```python
from build123d import *

# Parameters (mm, degrees)
ESQUISSE1_W                  = 40
ESQUISSE1_H                  = 85
BOSS_EXTRU_1_DEPTH           = 45
ESQUISSE2_W                  = 38.25
ESQUISSE2_H                  = 38.25
ENL_V_MAT_EXTRU_1_DEPTH      = 41.1
ESQUISSE3_W                  = 42
ESQUISSE3_H                  = 22
ENL_V_MAT_EXTRU_2_DEPTH      = 105.16333328
ESQUISSE4_R                  = 18.25625
ENL_V_MAT_EXTRU_3_DEPTH      = 42
ENL_V_MAT_EXTRU_4_DEPTH      = 104.048532255
ENL_V_MAT_EXTRU_4_DEPTH_BACK = 104.048532255
ESQUISSE5_R                  = 11
ESQUISSE6_R                  = 1.625
ENL_V_MAT_EXTRU_5_DEPTH      = 103.902866821
ENL_V_MAT_EXTRU_6_DEPTH      = 103.75038017
ENL_V_MAT_EXTRU_6_DEPTH_BACK = 103.75038017
ESQUISSE7_R                  = 4.065
ESQUISSE8_W                  = 5
ESQUISSE8_H                  = 21.25625
ENL_V_MAT_EXTRU_7_DEPTH      = 105.16333328


with BuildPart() as part:
    # Esquisse1 → Boss.-Extru.1 (new body)
    with BuildSketch(Plane.XY):
        with Locations((20, 42.5)):
            Rectangle(ESQUISSE1_W, ESQUISSE1_H)
    extrude(amount=BOSS_EXTRU_1_DEPTH)

    # Esquisse2 → Enlèv. mat.-Extru.1 (cut)
    with BuildSketch(Plane(origin=(40, 0, 0), x_dir=(0, 0, -1), z_dir=(1, 0, 0))):
        with Locations((-22.5, 19.125)):
            Rectangle(ESQUISSE2_W, ESQUISSE2_H)
    extrude(amount=-ENL_V_MAT_EXTRU_1_DEPTH, mode=Mode.SUBTRACT)

    # Esquisse3 → Enlèv. mat.-Extru.2 (cut, through all)
    with BuildSketch(Plane(origin=(0, 0, 45), x_dir=(0, 0, -1), z_dir=(1, 0, 0))):
        with Locations((24, 74)):
            Rectangle(ESQUISSE3_W, ESQUISSE3_H)
    extrude(amount=ENL_V_MAT_EXTRU_2_DEPTH, mode=Mode.SUBTRACT)

    # Esquisse4 → Enlèv. mat.-Extru.3 (cut)
    with BuildSketch(Plane.XY):
        with Locations((20, 63)):
            Circle(ESQUISSE4_R)
    extrude(amount=ENL_V_MAT_EXTRU_3_DEPTH, mode=Mode.SUBTRACT)

    # Esquisse5 → Enlèv. mat.-Extru.4 (cut, two sides: drawn at the far end of the back side and taken through both)
    with BuildSketch(Plane(origin=(37, 0, 0), x_dir=(-1, 0, 0), z_dir=(0, 0, -1)).offset(-ENL_V_MAT_EXTRU_4_DEPTH_BACK)):
        with Locations((17, 63)):
            Circle(ESQUISSE5_R)
    extrude(amount=ENL_V_MAT_EXTRU_4_DEPTH + ENL_V_MAT_EXTRU_4_DEPTH_BACK, mode=Mode.SUBTRACT)

    # Esquisse6 → Enlèv. mat.-Extru.5 (cut, through all)
    with BuildSketch(Plane(origin=(0, 0, 42), x_dir=(-1, 0, 0), z_dir=(0, 0, -1))):
        with Locations((-29.545941546, 72.545941546)):
            Circle(ESQUISSE6_R)
        with Locations((-29.545941546, 52.545941546)):
            Circle(ESQUISSE6_R)
        with Locations((-9.545941546, 52.545941546)):
            Circle(ESQUISSE6_R)
        with Locations((-9.545941546, 72.545941546)):
            Circle(ESQUISSE6_R)
    extrude(amount=-ENL_V_MAT_EXTRU_5_DEPTH, mode=Mode.SUBTRACT)

    # Esquisse7 → Enlèv. mat.-Extru.6 (cut, two sides: drawn at the far end of the back side and taken through both)
    with BuildSketch(Plane(origin=(0, 0, 41.625), x_dir=(-1, 0, 0), z_dir=(0, 0, -1)).offset(-ENL_V_MAT_EXTRU_6_DEPTH_BACK)):
        with Locations((-10, 18.4875)):
            Circle(ESQUISSE7_R)
        with Locations((-30, 18.4875)):
            Circle(ESQUISSE7_R)
    extrude(amount=ENL_V_MAT_EXTRU_6_DEPTH + ENL_V_MAT_EXTRU_6_DEPTH_BACK, mode=Mode.SUBTRACT)

    # Esquisse8 → Enlèv. mat.-Extru.7 (cut, through all)
    with BuildSketch(Plane.ZY):
        with Locations((2.5, 52.371875)):
            Rectangle(ESQUISSE8_W, ESQUISSE8_H)
    extrude(amount=-ENL_V_MAT_EXTRU_7_DEPTH, mode=Mode.SUBTRACT)


solid = part.part
```
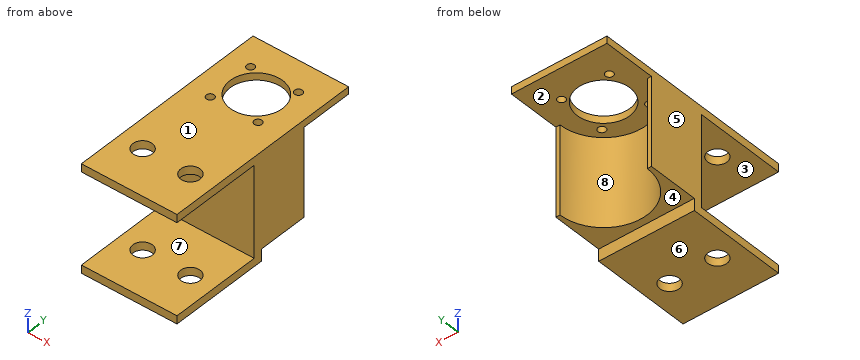
CAD build for the part. Positions are in the model's coordinates, mm. Face numbers are marked on the shaded views. A direction names the side the tool comes from. Coordinates: 2 decimals unless noted, no trailing zeros. Write each loop counter-clockwise with the first axis right and the second up, starting at its lowest first coordinate (ties: lowest second). Pieces come first, ordered by that corner, then holes. Notation, with made-up numbers: (65, 16.25) -> (78, 16.25) arc R30 cw to (78, 45.25) -> close; hole circle Ø4 at (49, 72). An arc over 180 degrees is marked (long way). Use CSV: the item, a comma, the result in double quotes. Start each with the question number.
Item 1: Drop flat-ended pins along their axis: P1, Ø8, axis at x = 11.5, y = 22, coming from the +Z side; P2, Ø8, axis at x = 29, z = 32, coming from the +Y side; P3, Ø12, axis at y = 72.5, z = 12, coming from the -X side; P4, Ø10.5, axis at x = 20.5, y = 49, coming from the -Z side. Give the stop position or say it passes through.
Item 2: Tool access for the marked faces 4, 5, 6, 7 and 8: list every direction of +Z, -Z, +X, -X, +Y, -Y with a clear straight run to the whole face (end or side of a thin tool).
Item 3: Band-saw the part on C-C, the plane x = 10. Give the number of separate pieces and of enclosed holes in the cut face, plus the area to 3 significant figures.
Item 4: Band-saw the part on D-D, the plane y = 20.5. Write the cut outline in (x, z) (3 decimals).
Item 5: Two-plate mould, pull along Z, no slides. Class the marked faces 1, 2 and 3: +Z half, -Z half, draft (parallel to the pull), parting line (faces both ways), or undercut.
Item 6: Band-saw the part on B-B, the plane y = 62. Write the cut outline in (x, z), plus the area to 3 significant figures.
Item 7: Band-saw the part on A-A, the plane x = 20. Write the cut outline in (y, z) (3 decimals), plus the area to 3 significant figures.
Item 8: Wall check: probe 1 along Z at (x, y) = (37.5, 34) (3 decimals); probe 2 along Y at (x, z) = (10, 0.9); probe 3 along Y at (x, z) = (20, 43). Give the ranges that are in metal, low to high.
Response values:
1,P1,"stops at z = 45"
1,P2,"stops at y = 50.18"
1,P3,"passes through"
1,P4,"stops at z = 5"
2,face 4,"-Z, +X, -X, +Y"
2,face 5,"+Z, -Z, -X, +Y, -Y"
2,face 6,"-Z, +X, -X, +Y, -Y"
2,face 7,"+X, -X, -Y"
2,face 8,"-Z, +Y"
3,separate pieces,"6"
3,enclosed holes,"0"
3,area,"665 mm2"
4,outline,"(0, 0) -> (6.468, 0) -> (6.468, 3.375) -> (0, 3.375) -> close; (0, 41.625) -> (6.468, 41.625) -> (6.468, 45) -> (0, 45) -> close; (13.532, 0) -> (26.468, 0) -> (26.468, 3.375) -> (13.532, 3.375) -> close; (13.532, 41.625) -> (26.468, 41.625) -> (26.468, 45) -> (13.532, 45) -> close; (33.532, 0) -> (40, 0) -> (40, 3.375) -> (33.532, 3.375) -> close; (33.532, 41.625) -> (40, 41.625) -> (40, 45) -> (33.532, 45) -> close"
5,face 1,"+Z half"
5,face 2,"-Z half"
5,face 3,"undercut"
6,outline,"(0, 5) -> (1.77, 5) -> (1.77, 42) -> (9.05, 42) -> (9.05, 45) -> (0, 45) -> close; (30.95, 42) -> (38.23, 42) -> (38.23, 5) -> (40, 5) -> (40, 45) -> (30.95, 45) -> close"
6,area,"185 mm2"
7,outline,"(0, 0) -> (41.744, 0) -> (41.744, 5) -> (44.744, 5) -> (44.744, 42) -> (52, 42) -> (52, 45) -> (0, 45) -> (0, 41.625) -> (38.25, 41.625) -> (38.25, 3.375) -> (0, 3.375) -> close; (74, 42) -> (85, 42) -> (85, 45) -> (74, 45) -> close"
7,area,"590 mm2"
8,probe 1,"z = 0 to 3.375, 41.625 to 45"
8,probe 2,"y = 0 to 14.42, 22.55 to 41.74"
8,probe 3,"y = 0 to 52, 74 to 85"
